Read the model definition and answer for the solid it produces. Units are mm, in the model's axes. A direction names the side the tool comes from. Coordinates: 2 decimals unless noted, no trailing zeros. Write each loop counter-clockwise with the first axis right and the second up, starting at its lowest first coordinate (ties: lowest second). Pieces come first, ordered by that corner, then holes.
Item 1: A tool of negligible diameter and unlimited length cuts with its end or side. For faces 4 (the face through (-11, 11.112, 0)), 5 (the face through (11.112, 9, 0)), 6 (the face through (0, 3, 23.019)), from which of +Z, -Z, +X, -X, +Y, -Y can it reach the whole face along a straight path? Write none if from no direction.
Item 2: Straight lines are drawn through the part: probe 1 along Z at (x, y) = (1, 1.5); probe 2 along X at (y, z) = (6.5, 4); probe 3 along Z at (x, y) = (-2, 8.5). For each, find the intervals that lie inside material, in ascending order.
Item 3: Section D-D (x = 20) is taken. Give the vertices of the cut face in (y, z), then the cut area to 3 significant figures.
Item 4: Section A-A (y = 4.5) is taken. Give the vertices of the cut face in (x, z).
Item 5: Section B-B (x = 0) is taken. Give the vertices of the cut face in (y, z), then the cut area to 3 significant figures.
Item 6: This flat-tipped pin is pushed along its axis until it touches: P1, Ø0.8, axis at x = 24.5, z = -13, coming from the +Y side (3 decimals). Where does it stop, or does it pass through?
Item 7: Determine the mould class of faces 1 (the face through (25.4, 5, 0)), 2 (the face through (23.812, 8, 0)), 3 (the face through (25, 9.525, 0)) for opening direction X: released by +X, released by -X, zero draft, split by the parting line, or undercut.
Autodesk Inventor part; units mm, degrees
ref_plane "YZ Plane" through (0, 0, 0) normal (1, 0, 0) x (0, 1, 0)
ref_plane "XZ Plane" through (0, 0, 0) normal (0, 1, 0) x (-1, 0, 0)
ref_plane "XY Plane" through (0, 0, 0) normal (0, 0, 1) x (1, 0, 0)
sketch "Sketch1" plane through (0, 0, 0) normal (0, 1, 0) x (-1, 0, 0)
  line L0 (-25.4, 31.75) -> (25.4, 31.75)
  line L1 (25.4, 31.75) -> (25.4, -31.75)
  line L2 (25.4, -31.75) -> (-25.4, -31.75)
  line L3 (-25.4, -31.75) -> (-25.4, 31.75)
  line L4 (-25.4, 31.75) -> (25.4, -31.75) construction
  line L5 (25.4, 31.75) -> (-25.4, -31.75) construction
  line L6 (0, 31.75) -> (0, -31.75) construction
  line L7 (-0.7937, -17.4625) -> (0.7938, -17.4625) construction
  line L8 (-0.7937, -23.0187) -> (0.7938, -23.0187)
  line L9 (0.7938, -11.9063) -> (-0.7937, -11.9063)
  arc A0 (-0.7937, -11.9063) -> (-0.7937, -23.0187) centre (-0.7937, -17.4625) ccw
  arc A1 (0.7938, -23.0187) -> (0.7938, -11.9063) centre (0.7938, -17.4625) ccw
  line L10 (25.4, 0) -> (-25.4, 0) construction
  line L11 (-0.7937, 17.4625) -> (0.7937, 17.4625) construction
  line L12 (-0.7938, 23.0187) -> (0.7937, 23.0187)
  line L13 (0.7938, 11.9063) -> (-0.7937, 11.9063)
  arc A2 (-0.7938, 23.0187) -> (-0.7937, 11.9063) centre (-0.7937, 17.4625) ccw
  arc A3 (0.7938, 11.9063) -> (0.7937, 23.0187) centre (0.7937, 17.4625) ccw
  circle A4 centre (0, 17.4625) radius 5.5562
  circle A5 centre (0, -17.4625) radius 5.5562
  point P0 (0, 0)
  point P1 (0, 0)
  point P2 (0, -11.9063)
  point P3 (0, -23.0187)
  point P4 (0, 11.9063)
  point P5 (0, 23.0187)
  dimension "d0" = 50.8
  dimension "d1" = 63.5
  dimension "d2" = 0.7937
  dimension "d3" = 11.1125
  dimension "d4" = 17.4625
extrude "Extrusion1" add sketch "Sketch1" along normal blind 11.1125 contours L0 L1 L2 L3 | A0 L9 A5 L8 | A5 L9 A1 L8 | L12 A4 L13 A2 | L12 A3 L13 A4
sketch "Sketch2" plane through (0, 11.1125, 0) normal (0, 1, 0) x (1, 0, 0)
  line L0 (25.4, 31.75) -> (-25.4, 31.75)
  line L1 (-25.4, -31.75) -> (25.4, -31.75)
  line L2 (23.8125, 31.75) -> (11.1125, 31.75)
  line L3 (11.1125, 31.75) -> (11.1125, -31.75)
  line L4 (11.1125, -31.75) -> (23.8125, -31.75)
  line L5 (23.8125, -31.75) -> (23.8125, 31.75)
  line L6 (25.4, -31.75) -> (25.4, 31.75)
  point P0 (0, 0)
  point P1 (23.8125, -31.75)
  dimension "d7" = 12.7
  dimension "d8" = 1.5875
extrude "Extrusion3" cut sketch "Sketch2" against normal blind 1.5875 contours L6 L1 L5 L0
chamfer "Chamfer1" distance 4.7625 angle 49 2 edges at (0, 11.1125, 23.0188) (0, 11.1125, -23.0188) measured on face at (-18.6651, 11.1125, -5.1641)
extrude "Extrusion4" cut sketch "Sketch2" against normal blind 4.7625 contours L5 L1 L3 L0
extrude "Extrusion5" cut sketch "Sketch1" along normal blind 7.9375 contours A0 L9 A5 L8 | A5 L9 A1 L8 | A5 | L12 A4 L13 A2 | L12 A3 L13 A4 | A4
properties part number "Jaw" material "Aluminum 6061"
Established:
1. face 4: +Z, -Z, +X, -X, +Y
1. face 5: +Z, -Z, +Y
1. face 6: +Y, -Y
2. probe 1: z = -31.75 to -23.01, -11.91 to 11.91, 23.01 to 31.75
2. probe 2: x = -25.4 to 11.11, 23.81 to 25.4
2. probe 3: z = -31.75 to -25.26, -9.67 to 9.67, 25.26 to 31.75
3. outline: (0, -31.75) - (6.35, -31.75) - (6.35, 31.75) - (0, 31.75) - close
3. area: 403 mm2
4. outline: (-25.4, -31.75) - (25.4, -31.75) - (25.4, 31.75) - (-25.4, 31.75) - close; hole (-0.79, -23.02) - (0.79, -23.02) arc R5.56 ccw to (0.79, -11.91) - (-0.79, -11.91) arc R5.56 ccw to start; hole (-0.79, 11.91) - (0.79, 11.91) arc R5.56 ccw to (0.79, 23.02) - (-0.79, 23.02) arc R5.56 ccw to start
5. outline: (0, -31.75) - (11.11, -31.75) - (11.11, -27.78) - (5.63, -23.02) - (0, -23.02) - close; (0, -11.91) - (5.63, -11.91) - (11.11, -7.14) - (11.11, 7.14) - (5.63, 11.91) - (0, 11.91) - close; (0, 23.02) - (5.63, 23.02) - (11.11, 27.78) - (11.11, 31.75) - (0, 31.75) - close
5. area: 406 mm2
6. P1: stops at y = 9.525
7. face 1: released by +X
7. face 2: undercut
7. face 3: zero draft
